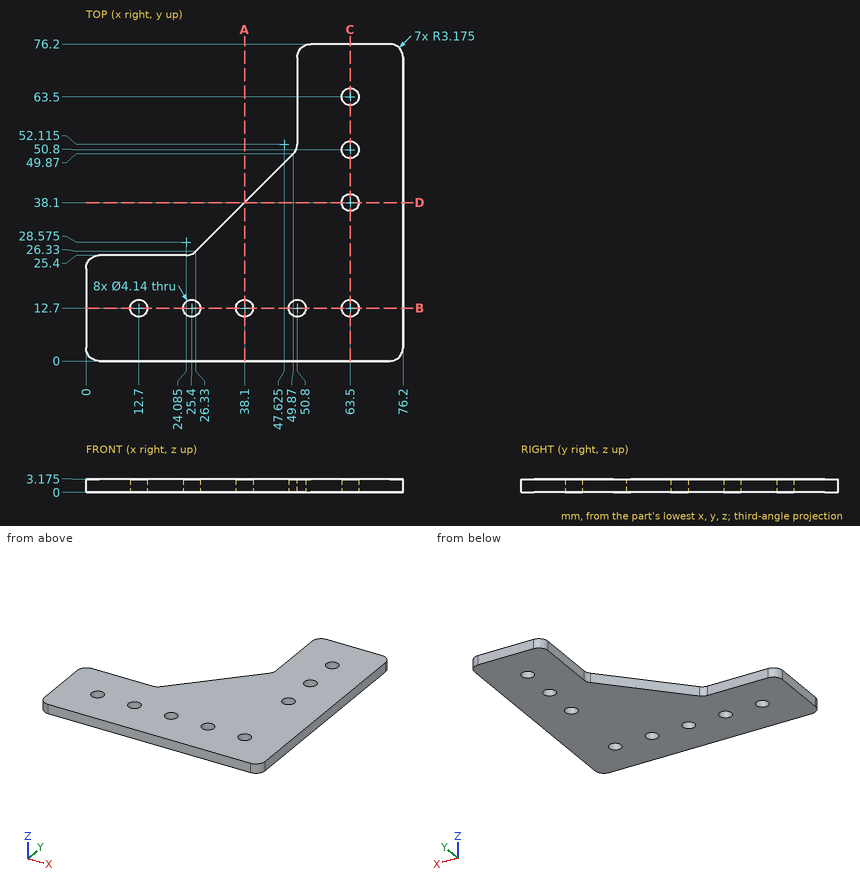
Could you check a few things on this drawing? It's one solid part, dimensions in mm from its lowest x, y, z. Give positions to 0.01 mm unless a question says otherwise; leave off trailing zeros. Order: outer loops, then holes, each group sorted by start corner. A loop starts at its lowest first (then second) coordinate and runs counter-clockwise, first axis right, second up. Notation, with made-up numbers: (16, 22.5) -> (73, 22.5) arc R27 cw to (73, 41.5) -> close; hole circle Ø6 at (43.25, 79.25). An arc over 180 degrees is marked (long way). Answer in a Markdown table with one row per item. Add a question column.
Item 1: Please list where these lines run through material, in increasing order: probe 1 along X at (y, z) = (12.7, 2.15); probe 2 along Y at (x, z) = (63.5, 0.85); probe 3 along Y at (x, z) = (12.7, 1.55).
Item 2: Imagine slicing it at C-C (x = 63.5). List the corners of the cut face in (y, z) for me (1 decimal).
Item 3: Imagine slicing it at B-B (y = 12.7). List the corners of the cut face in (x, z) for me (1 decimal), and give its area (3 significant figures).
Item 4: Imagine slicing it at A-A (x = 38.1). List the corners of the cut face in (y, z) for me (1 decimal).
Item 5: Imagine slicing it at D-D (y = 38.1). List the corners of the cut face in (x, z) for me (1 decimal), and give its area (3 significant figures).
Item 6: I'm going to push a flat-ended pin straight in: P1, Ø10, axis at x = 43.5, y = 41.5, coming from the -Z side. Where does the tip first touch, or does it pass through?
Result:
| question | item | result |
|---|---|---|
| 1 | probe 1 | 0 to 10.63, 14.77 to 23.33, 27.47 to 36.03, 40.17 to 48.73, 52.87 to 61.43, 65.57 to 76.2 |
| 1 | probe 2 | 0 to 10.63, 14.77 to 36.03, 40.17 to 48.73, 52.87 to 61.43, 65.57 to 76.2 |
| 1 | probe 3 | 0 to 10.63, 14.77 to 25.4 |
| 2 | outline | (0, 0) -> (10.6, 0) -> (10.6, 3.2) -> (0, 3.2) -> close; (14.8, 0) -> (36, 0) -> (36, 3.2) -> (14.8, 3.2) -> close; (40.2, 0) -> (48.7, 0) -> (48.7, 3.2) -> (40.2, 3.2) -> close; (52.9, 0) -> (61.4, 0) -> (61.4, 3.2) -> (52.9, 3.2) -> close; (65.6, 0) -> (76.2, 0) -> (76.2, 3.2) -> (65.6, 3.2) -> close |
| 3 | outline | (0, 0) -> (10.6, 0) -> (10.6, 3.2) -> (0, 3.2) -> close; (14.8, 0) -> (23.3, 0) -> (23.3, 3.2) -> (14.8, 3.2) -> close; (27.5, 0) -> (36, 0) -> (36, 3.2) -> (27.5, 3.2) -> close; (40.2, 0) -> (48.7, 0) -> (48.7, 3.2) -> (40.2, 3.2) -> close; (52.9, 0) -> (61.4, 0) -> (61.4, 3.2) -> (52.9, 3.2) -> close; (65.6, 0) -> (76.2, 0) -> (76.2, 3.2) -> (65.6, 3.2) -> close |
| 3 | area | 176 mm2 |
| 4 | outline | (0, 0) -> (10.6, 0) -> (10.6, 3.2) -> (0, 3.2) -> close; (14.8, 0) -> (38.1, 0) -> (38.1, 3.2) -> (14.8, 3.2) -> close |
| 5 | outline | (38.1, 0) -> (61.4, 0) -> (61.4, 3.2) -> (38.1, 3.2) -> close; (65.6, 0) -> (76.2, 0) -> (76.2, 3.2) -> (65.6, 3.2) -> close |
| 5 | area | 108 mm2 |
| 6 | P1 | z = 0 |
